Geometry check sheet. Reference: the model listing, model coordinates, mm. A direction names the side the tool comes from. Round coordinates to 2 decimals unless told otherwise and drop trailing zeros. Order: outer loops, then holes, each group sorted by start corner. A loop starts at its lowest first (then second) coordinate and runs counter-clockwise, first axis right, second up. Notation, with made-up numbers: (69.25, -16.5) - (112.25, -16.5) arc R25 ccw to (112.25, 14.5) - close; hole circle Ø9 at (44, -34.75). An arc over 180 degrees is marked (long way). Use a Markdown table: item, result. Add a question column.
(1) Access from +Z, -Z, +X, -X, +Y, -Y to the whole of each face (thin tool, end or side, straight path). Record for faces 1 (the face through (-30.666, 5.5, -20.5)), 2 (the face through (-20.291, 7, -25)), 3 (the face through (-36.541, 1, -25)), 4 (the face through (-29, 4, -29.09)), 5 (the face through (-20, 6.4, -25)).
(2) Section check A-A on z = -24. Record the boundary of the cut face in (x, y), then the cut area to 3 significant figures.
(3) Section check C-C on x = -32.25. Record the boundary of the cut face in (y, z), then the cut area to 3 significant figures.
(4) Section check D-D on z = -22. Record the boundary of the cut face in (x, y), then the cut area to 3 significant figures.
(5) Mould release check, pull along Z, two halves, no side actions. Record for faces 6 (the face through (-29, 1, -20.09)), 7 (the face through (-20, 3, -22.34)), 8 (the face through (-37.341, 7, -25)): released by +Z, released by -Z, zero draft, split by the parting line, or undercut.
(6) Gauge pin test, flat ends, axial feed: P1, Ø0.6, axis at y = 1, z = -25.5, coming from the +X side; P2, Ø2, axis at y = 5, z = -25.5, coming from the -X side. Record the tip position at first contact, or that the pin passes through.
(7) Thickness scan on line 1 along Z through (x, y) = (-24.5, 5.5); line 2 along X through (y, z) = (6.5, -25.5); line 3 along Z through (x, y) = (-34.75, 2.5). Record the ranges inside material, lowest first. Write a range as [from, to].
(8) Section check B-B on y = -1.5. Give the number of separate pieces and of enclosed holes in the cut face, then the cut area to 3 significant figures.
```python
from build123d import *

# Parameters (mm, degrees)
SKETCH1_W           = 17.85
SKETCH1_H           = 9
BOSS_EXTRUDE1_DEPTH = 9.1
SKETCH2_W           = 16.25
SKETCH2_H           = 7.4
CUT_EXTRUDE1_DEPTH  = 7.1
SKETCH2_3_W         = 0.8
SKETCH2_3_H         = 0.8
BOSS_EXTRUDE2_DEPTH = 12.5
SKETCH3_W           = 4.5
SKETCH3_H           = 7.1
CUT_EXTRUDE2_DEPTH  = 2.1
SKETCH5_W           = 4.5
SKETCH5_H           = 6.4
CUT_EXTRUDE3_DEPTH  = 0.8
SKETCH6_W           = 4.5
SKETCH6_H           = 6.4
CUT_EXTRUDE4_DEPTH  = 0.8


with BuildPart() as part:
    # Sketch1 → Boss-Extrude1 (new body)
    with BuildSketch(Plane(origin=(0, 0, 0), x_dir=(1, 0, 0), z_dir=(0, 1, 0))):
        with Locations((-28.415572658, 24.590099186)):
            Rectangle(SKETCH1_W, SKETCH1_H)
    extrude(amount=BOSS_EXTRUDE1_DEPTH)

    # Sketch2 → Cut-Extrude1 (cut)
    with BuildSketch(Plane(origin=(0, 9.1, 0), x_dir=(1, 0, 0), z_dir=(0, 1, 0))):
        with Locations((-28.415572658, 24.590099186)):
            Rectangle(SKETCH2_W, SKETCH2_H)
    extrude(amount=-CUT_EXTRUDE1_DEPTH, mode=Mode.SUBTRACT)

    # Sketch2<3> → Boss-Extrude2 (add)
    with BuildSketch(Plane(origin=(0, 9.1, 0), x_dir=(1, 0, 0), z_dir=(0, 1, 0))):
        with Locations((-29.685572658, 23.320099186)):
            Rectangle(SKETCH2_3_W, SKETCH2_3_H)
        with Locations((-27.145572658, 23.320099186)):
            Rectangle(SKETCH2_3_W, SKETCH2_3_H)
        with Locations((-24.605572658, 23.320099186)):
            Rectangle(SKETCH2_3_W, SKETCH2_3_H)
        with Locations((-27.145572658, 25.860099186)):
            Rectangle(SKETCH2_3_W, SKETCH2_3_H)
        with Locations((-24.605572658, 25.860099186)):
            Rectangle(SKETCH2_3_W, SKETCH2_3_H)
        with Locations((-29.685572658, 25.860099186)):
            Rectangle(SKETCH2_3_W, SKETCH2_3_H)
        with Locations((-32.225572658, 23.320099186)):
            Rectangle(SKETCH2_3_W, SKETCH2_3_H)
        with Locations((-32.225572658, 25.860099186)):
            Rectangle(SKETCH2_3_W, SKETCH2_3_H)
    extrude(amount=-BOSS_EXTRUDE2_DEPTH)

    # Sketch3 → Cut-Extrude2 (cut)
    with BuildSketch(Plane.XY.offset(-20.090099186)):
        with Locations((-28.415572658, 5.55)):
            Rectangle(SKETCH3_W, SKETCH3_H)
    extrude(amount=-CUT_EXTRUDE2_DEPTH, mode=Mode.SUBTRACT)

    # Sketch5 → Cut-Extrude3 (cut)
    with BuildSketch(Plane.ZY.offset(37.340572658)):
        with Locations((-24.590099186, 3.2)):
            Rectangle(SKETCH5_W, SKETCH5_H)
    extrude(amount=-CUT_EXTRUDE3_DEPTH, mode=Mode.SUBTRACT)

    # Sketch6 → Cut-Extrude4 (cut)
    with BuildSketch(Plane(origin=(-19.490572658, 0, 0), x_dir=(0, 0, -1), z_dir=(1, 0, 0))):
        with Locations((24.590099186, 3.2)):
            Rectangle(SKETCH6_W, SKETCH6_H)
    extrude(amount=-CUT_EXTRUDE4_DEPTH, mode=Mode.SUBTRACT)


solid = part.part
```
Check sheet entries:
| question | item | result |
|---|---|---|
| 1 | face 1 | +Z, +Y |
| 1 | face 2 | +Y |
| 1 | face 3 | -X, -Y |
| 1 | face 4 | -Z, +X, -X, +Y, -Y |
| 1 | face 5 | +X, -Y |
| 2 | outline | (-37.34, 6.4) - (-36.54, 6.4) - (-36.54, 9.1) - (-37.34, 9.1) - close; (-36.54, 0) - (-20.29, 0) - (-20.29, 2) - (-36.54, 2) - close; (-20.29, 6.4) - (-19.49, 6.4) - (-19.49, 9.1) - (-20.29, 9.1) - close |
| 2 | area | 36.8 mm2 |
| 3 | outline | (-3.4, -26.26) - (0, -26.26) - (0, -29.09) - (9.1, -29.09) - (9.1, -28.29) - (2, -28.29) - (2, -26.26) - (9.1, -26.26) - (9.1, -25.46) - (2, -25.46) - (2, -23.72) - (9.1, -23.72) - (9.1, -22.92) - (2, -22.92) - (2, -20.89) - (9.1, -20.89) - (9.1, -20.09) - (0, -20.09) - (0, -22.92) - (-3.4, -22.92) - (-3.4, -23.72) - (0, -23.72) - (0, -25.46) - (-3.4, -25.46) - close |
| 3 | area | 46.2 mm2 |
| 4 | outline | (-37.34, 0) - (-19.49, 0) - (-19.49, 9.1) - (-20.29, 9.1) - (-20.29, 2) - (-36.54, 2) - (-36.54, 9.1) - (-37.34, 9.1) - close |
| 4 | area | 47.1 mm2 |
| 5 | face 6 | released by +Z |
| 5 | face 7 | undercut |
| 5 | face 8 | zero draft |
| 6 | P1 | stops at x = -20.29 |
| 6 | P2 | stops at x = -32.63 |
| 7 | line 1 | z = [-29.09, -28.29], [-26.26, -25.46], [-23.72, -22.92], [-20.89, -20.09] |
| 7 | line 2 | x = [-37.34, -36.54], [-32.63, -31.83], [-30.09, -29.29], [-27.55, -26.75], [-25.01, -24.21], [-20.29, -19.49] |
| 7 | line 3 | z = [-29.09, -28.29], [-20.89, -20.09] |
| 8 | separate pieces | 8 |
| 8 | enclosed holes | 0 |
| 8 | area | 5.12 mm2 |
